Autodesk Inventor part; units mm, degrees
ref_plane "Work Plane1" through (29, 0, 0) normal (0, -1, 0) x (1, 0, 0)
ref_plane "YZ Plane" through (0, 0, 0) normal (1, 0, 0) x (0, 1, 0)
ref_plane "XZ Plane" through (0, 0, 0) normal (0, 1, 0) x (-1, 0, 0)
sketch "Szkic1" plane through (0, 0, 0) normal (0, 0, 1) x (1, 0, 0)
  line L0 (0.1667, 0) -> (8, 0)
  line L1 (8, 0) -> (8, 1.5)
  line L2 (8, 1.5) -> (1.5, 1.5)
  line L3 (1.5, 1.5) -> (1.1932, 1.5)
  line L4 (1.1932, 1.5) -> (0, 1.5)
  line L5 (0, 1.5) -> (0, 2.75)
  line L6 (0, 2.75) -> (-2, 2.75)
  line L7 (-2, 2.75) -> (-2, 1.1547)
  line L8 (-2, 1.1547) -> (-0.5, 1.1547)
  line L9 (-0.5, 1.1547) -> (0.1667, 0)
  line L10 (-4, 0) -> (10, 0)
  line L11 (0, -0.55) -> (0, 3.3)
  line L12 (1.5, 1.5) -> (0, 1.5) construction
  dimension "d1" = 6.5
  dimension "d2" = 0.3068
  dimension "d3" = 2
  dimension "d4" = 1.5
  dimension "d5" = 60
  dimension "d6" = 3
  dimension "d7" = 3
  dimension "d8" = 2.3094
  dimension "d9" = 5.5
  dimension "d26" = 8
revolve "Bryła" add sketch "Szkic1" angle 360 about axis through (0.1667, 0, 0) along (1, 0, 0) contours L9 L11 L4 L3 L2 L1 L0 | L9 L8 L7 L6 L5 L11
sketch "Szkic2" plane through (-2, 0, 0) normal (-1, 0, 0) x (0, 0, 1)
  circle A0 centre (0, 0) radius 1.1547
  line L0 (0, -3.85) -> (0, 3.85)
  line L1 (-3.85, 0) -> (3.85, 0)
  line L2 (1.1547, 0) -> (0.5774, -1)
  line L3 (0.5774, -1) -> (-0.5774, -1)
  line L4 (-0.5774, -1) -> (-1.1547, 0)
  line L5 (-1.1547, 0) -> (-0.5774, 1)
  line L6 (-0.5774, 1) -> (0.5774, 1)
  line L7 (0.5774, 1) -> (1.1547, 0)
  point P0 (0, 0)
extrude "Szczelina" add sketch "Szkic2" against normal up to next contours L7 A0 | A0 L2 | L6 L0 A0 | A0 L0 L3 | L0 L6 A0 | A0 L3 L0 | L4 A0 | A0 L5
fillet "Zaokrąglenie1" radius 0.3 1 edges at (-2, -2.75, 0)
thread "Gwint"
chamfer "Faza1" distance 0.3067 distance2 0.3067 1 edges at (8, -1.5, 0) measured on face at (8, 0.5539, 0.4443)
ref_plane "Work Plane1" through (29, 0, 0) normal (0, -1, 0) x (1, 0, 0)
fillet "Fillet2" radius 0.1 1 edges at (0, -1.5, 0)
equation "\"d1\" = GEL"
equation "\"d3\" = KOH"
equation "\"d4\" = INTI"
equation "\"d6\" = GD"
equation "\"d7\" = BDM"
equation "\"d8\" = 1.1547 * SW"
equation "\"d9\" = KOD"
equation "\"d26\" = NLG"
equation "\"d30\" = R"
equation "\"d17\" = RR"
equation "\"d13\" = GEL"
equation "\"d15\" = -0.5 * SPD + 0.5 * GD"
equation "\"d16\" = GUL"
equation "\"GD\" = NND"
equation "\"NLG\" = 8"
equation "\"GEL\" = 6.5"
equation "\"KOD\" = 5.5"
equation "\"KOH\" = 2"
equation "\"INTI\" = 1.5"
equation "\"GAL\" = 0.61345 * PTC"
equation "\"GUL\" = 0.61345 * PTC"
equation "\"BDM\" = NND"
equation "\"SW\" = 2"
equation "\"RR\" = 0.3"
equation "\"SPD\" = NND - 1.2269 * PTC"
equation "\"R\" = 0.1"
equation "\"TOA\" = 30deg"
equation "\"GD1\" = THREADDIA - 1.2269 * PTC"
equation "\"THREADDIA\" = 3"
equation "\"FAWI\" = 45deg"
equation "\"ANG\" = 120deg"
equation "\"PTC\" = 0.5"
equation "\"NND\" = 3"
equation "\"E0\" = 1.155 * SW"
properties part number "DIN 7984 - M3 x 8" material "Stal, miękka"
Geometry: final body of the model. Coordinates: model frame, mm. A direction names the side the tool comes from. Coordinates: 2 decimals unless noted, no trailing zeros. Order: outer loops, then holes, each group sorted by start corner. A loop starts at its lowest first (then second) coordinate and runs counter-clockwise, first axis right, second up. Notation, with made-up numbers: (86, 47) - (102, 47) arc R16 ccw to (102, 64) - close; hole circle Ø1 at (-27.75, 31.25). An arc over 180 degrees is marked (long way). Use one line per item in the form item = value.
1) Mould query, pull axis Z, two halves, no side actions, for faces 4 (the face through (0, 2, 0)), 5 (the face through (-0.862, -0.596, 2.685)), 6 (the face through (-1.22, 0.51, 0.86)). Classes: +Z half, -Z half, draft (parallel to the pull), parting line (faces both ways), or undercut.
Solutions:
face_4 = draft
face_5 = parting line
face_6 = undercut
2) Pin query (flat end, axial travel): pin 1 (2 mm diameter, centred on x = 6.5, y = 0, fed in from +Z); pin 2 (1.5 mm diameter, centred on x = -0.5, y = 0.5, fed in from +Z). Return the tip coordinate at first contact, or that it passes through.
Solutions:
pin_1 = 1.5
pin_2 = 2.75
3) Set-up query: faces 1 (the face through (-1, -1, 0)), 2 (the face through (3.84, -1.5, -0.07)), 3 (the face through (-2, -1, 1)). Return all of +Z, -Z, +X, -X, +Y, -Y with unobstructed straight access to the full face (end or side cutting, diameter ignored); none if empty.
Solutions:
face_1 = -X
face_2 = +X
face_3 = +Z, -Z, -X, +Y, -Y
4) Ray query, L1, parallel to X at y = 0.4, z = 1.75; L2, parallel to X at y = 0, z = 1; L3, parallel to Y at x = -1.25, z = 0.8. Return the intervals inside material, ascending.
Solutions:
L1 = -2 to 0
L2 = -0.41 to 8
L3 = -2.63 to -0.61, 0.61 to 2.63
5) Section A-A (x = 1.25). Return loops of the section in (y, z), then the cut area to 3 significant figures.
Solutions:
outline = circle Ø3 at (0, 0)
area = 7.07 mm^2
